The listing builds one solid part. Answer for the finished solid, in the listing's coordinates (mm). Coordinates: 2 decimals unless noted, no trailing zeros. Write item = value, one per line. Start each with the question number.
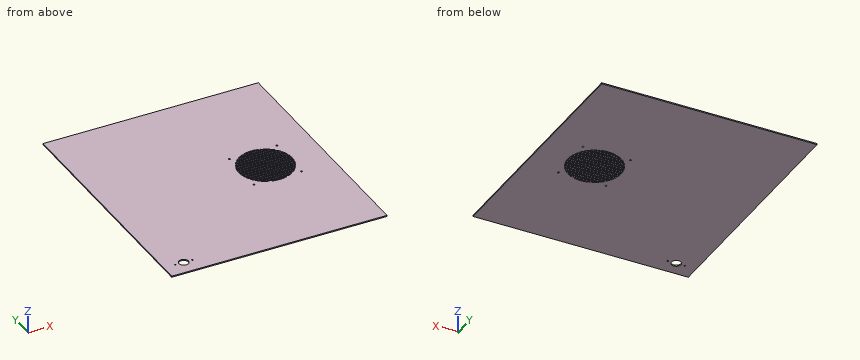
```python
from build123d import *

# Parameters (mm, degrees)
SKICA1_W                = 565
SKICA1_H                = 645
SKICA1_R                = 2
SKICA1_R_2              = 12.5
SKICA1_R_3              = 2.3
P_IDAT_VYSUNUT_M1_DEPTH = 3


with BuildPart() as part:
    # Skica1 → Přidat vysunutím1 (new body)
    with BuildSketch(Plane.XY):
        Rectangle(SKICA1_W, SKICA1_H)
        with BuildLine():
            Line((177.343477787, -53.75), (87.656522213, -53.75))
            ThreePointArc((87.656522213, -53.75), (83.661766134, -50.148049941), (79.955376108, -46.25))
            Line((79.955376108, -46.25), (185.044623892, -46.25))
            ThreePointArc((185.044623892, -46.25), (181.338233866, -50.148049941), (177.343477787, -53.75))
        make_face(mode=Mode.SUBTRACT)
        with BuildLine():
            Line((90.835416719, -56.25), (174.164583281, -56.25))
            ThreePointArc((174.164583281, -56.25), (167.987274157, -60.337827048), (161.412583766, -63.75))
            Line((161.412583766, -63.75), (103.587416234, -63.75))
            ThreePointArc((103.587416234, -63.75), (97.012725843, -60.337827048), (90.835416719, -56.25))
        make_face(mode=Mode.SUBTRACT)
        with Locations((-252.5, -282.5)):
            Circle(SKICA1_R, mode=Mode.SUBTRACT)
        with Locations((-230, -282.5)):
            Circle(SKICA1_R_2, mode=Mode.SUBTRACT)
        with Locations((-207.5, -282.5)):
            Circle(SKICA1_R, mode=Mode.SUBTRACT)
        with BuildLine():
            ThreePointArc((192.382697835, -36.25), (189.885872046, -40.085679357), (187.143732486, -43.75))
            Line((187.143732486, -43.75), (77.856267514, -43.75))
            ThreePointArc((77.856267514, -43.75), (75.114127954, -40.085679357), (72.617302165, -36.25))
            Line((72.617302165, -36.25), (192.382697835, -36.25))
        make_face(mode=Mode.SUBTRACT)
        with BuildLine():
            ThreePointArc((197.391736762, -26.25), (195.720425822, -30.052915979), (193.82648286, -33.75))
            Line((193.82648286, -33.75), (71.17351714, -33.75))
            ThreePointArc((71.17351714, -33.75), (69.279574178, -30.052915979), (67.608263238, -26.25))
            Line((67.608263238, -26.25), (197.391736762, -26.25))
        make_face(mode=Mode.SUBTRACT)
        with BuildLine():
            ThreePointArc((200.587719157, -16.25), (199.572689903, -20.031332187), (198.347835955, -23.75))
            Line((198.347835955, -23.75), (66.652164045, -23.75))
            ThreePointArc((66.652164045, -23.75), (65.427310097, -20.031332187), (64.412280843, -16.25))
            Line((64.412280843, -16.25), (200.587719157, -16.25))
        make_face(mode=Mode.SUBTRACT)
        with BuildLine():
            ThreePointArc((202.220423837, -6.25), (201.779911608, -10.014681604), (201.136269566, -13.75))
            Line((201.136269566, -13.75), (63.863730434, -13.75))
            ThreePointArc((63.863730434, -13.75), (63.220088392, -10.014681604), (62.779576163, -6.25))
            Line((62.779576163, -6.25), (202.220423837, -6.25))
        make_face(mode=Mode.SUBTRACT)
        with BuildLine():
            Line((202.3994814, -3.75), (62.6005186, -3.75))
            ThreePointArc((62.6005186, -3.75), (62.5, 0), (62.6005186, 3.75))
            Line((62.6005186, 3.75), (202.3994814, 3.75))
            ThreePointArc((202.3994814, 3.75), (202.5, 0), (202.3994814, -3.75))
        make_face(mode=Mode.SUBTRACT)
        with BuildLine():
            ThreePointArc((201.136269566, 13.75), (201.779911608, 10.014681604), (202.220423837, 6.25))
            Line((202.220423837, 6.25), (62.779576163, 6.25))
            ThreePointArc((62.779576163, 6.25), (63.220088392, 10.014681604), (63.863730434, 13.75))
            Line((63.863730434, 13.75), (201.136269566, 13.75))
        make_face(mode=Mode.SUBTRACT)
        with BuildLine():
            ThreePointArc((198.347835955, 23.75), (199.572689903, 20.031332187), (200.587719157, 16.25))
            Line((200.587719157, 16.25), (64.412280843, 16.25))
            ThreePointArc((64.412280843, 16.25), (65.427310097, 20.031332187), (66.652164045, 23.75))
            Line((66.652164045, 23.75), (198.347835955, 23.75))
        make_face(mode=Mode.SUBTRACT)
        with BuildLine():
            ThreePointArc((193.82648286, 33.75), (195.720425822, 30.052915979), (197.391736762, 26.25))
            Line((197.391736762, 26.25), (67.608263238, 26.25))
            ThreePointArc((67.608263238, 26.25), (69.279574178, 30.052915979), (71.17351714, 33.75))
            Line((71.17351714, 33.75), (193.82648286, 33.75))
        make_face(mode=Mode.SUBTRACT)
        with BuildLine():
            ThreePointArc((187.143732486, 43.75), (189.885872046, 40.085679357), (192.382697835, 36.25))
            Line((192.382697835, 36.25), (72.617302165, 36.25))
            ThreePointArc((72.617302165, 36.25), (75.114127954, 40.085679357), (77.856267514, 43.75))
            Line((77.856267514, 43.75), (187.143732486, 43.75))
        make_face(mode=Mode.SUBTRACT)
        with BuildLine():
            ThreePointArc((177.343477787, 53.75), (181.338233866, 50.148049941), (185.044623892, 46.25))
            Line((185.044623892, 46.25), (79.955376108, 46.25))
            ThreePointArc((79.955376108, 46.25), (83.661766134, 50.148049941), (87.656522213, 53.75))
            Line((87.656522213, 53.75), (177.343477787, 53.75))
        make_face(mode=Mode.SUBTRACT)
        with BuildLine():
            ThreePointArc((161.412583766, 63.75), (167.987274157, 60.337827048), (174.164583281, 56.25))
            Line((174.164583281, 56.25), (90.835416719, 56.25))
            ThreePointArc((90.835416719, 56.25), (97.012725843, 60.337827048), (103.587416234, 63.75))
            Line((103.587416234, 63.75), (161.412583766, 63.75))
        make_face(mode=Mode.SUBTRACT)
        with Locations((194.75, 62.25)):
            Circle(SKICA1_R_3, mode=Mode.SUBTRACT)
        with BuildLine():
            ThreePointArc((109.89607335, 66.25), (132.5, 70), (155.10392665, 66.25))
            Line((155.10392665, 66.25), (109.89607335, 66.25))
        make_face(mode=Mode.SUBTRACT)
        with Locations((70.25, 62.25)):
            Circle(SKICA1_R_3, mode=Mode.SUBTRACT)
        with Locations((194.75, -62.25)):
            Circle(SKICA1_R_3, mode=Mode.SUBTRACT)
        with Locations((70.25, -62.25)):
            Circle(SKICA1_R_3, mode=Mode.SUBTRACT)
        with BuildLine():
            ThreePointArc((155.10392665, -66.25), (132.5, -70), (109.89607335, -66.25))
            Line((109.89607335, -66.25), (155.10392665, -66.25))
        make_face(mode=Mode.SUBTRACT)
    extrude(amount=P_IDAT_VYSUNUT_M1_DEPTH)


solid = part.part
```
1. A straight line is drawn through the part: L1, parallel to Y at x = -252.5, z = 0.75. Find the intervals that lie inside material, in ascending order. Write a range as [from, to].
2. This flat-tipped pin is pushed along its axis until it touches: pin 1 (15 mm diameter, centred on x = -230, y = -282.5, fed in from +Z). Where does it stop, or does it pass through?
3. The part is cut by section A-A, the plane z = 2.25. Count the separate pieces of the cut face and the enclosed holes in it, and give its area (3 significant figures).
Solution:
q1.L1 = [-322.5, -284.5], [-280.5, 322.5]
q2.pin_1 = through
q3.separate_pieces = 1
q3.enclosed_holes = 22
q3.area = 352,000 mm^2
